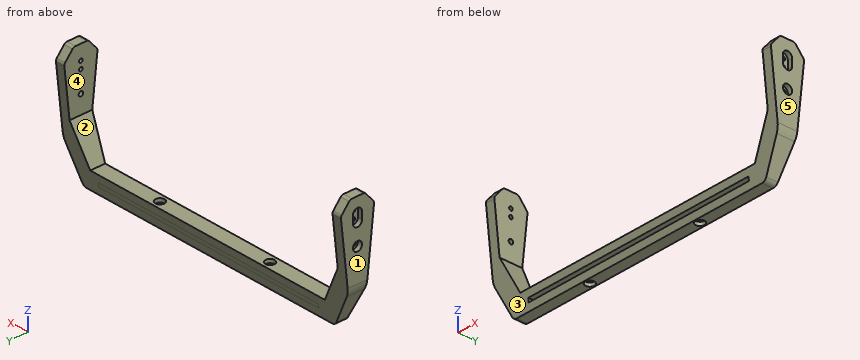
from build123d import *
from OCP.BRepFilletAPI import BRepFilletAPI_MakeChamfer

# Parameters (mm, degrees)
SKETCH4_R                       = 1
SKETCH4_R_2                     = 0.9999999999999998
SKETCH4_R_3                     = 1.250000000000001
BOSS_EXTRUDE1_DEPTH             = 5
BOSS_EXTRUDE2_START             = -79.75
BOSS_EXTRUDE2_DEPTH             = 159.5
BOSS_EXTRUDE3_REACH             = 103.717
SKETCH6_W                       = 14.25
SKETCH6_H                       = 2.1000000000000014
BOSS_EXTRUDE3_DIRECTION_2_REACH = 103.717
SKETCH11_R                      = 0.9999999999999983
CUT_EXTRUDE4_DEPTH              = 101.58679916039975
SKETCH12_R                      = 2.4999999999999982
SKETCH12_R_2                    = 2.500000000000002
CUT_EXTRUDE5_DEPTH              = 2
CUT_EXTRUDE6_START              = -2
SKETCH13_R                      = 2.4999999999999982
SKETCH13_R_2                    = 2.500000000000002
CUT_EXTRUDE6_DEPTH              = 2
CHAMFER3_SIZE                   = 10
CHAMFER3_SIZE2                  = 20
CHAMFER4_SIZE                   = 20
CHAMFER4_SIZE2                  = 10
BOSS_EXTRUDE4_START             = -65.5
BOSS_EXTRUDE4_DEPTH             = 131
SKETCH15_R                      = 2.4999999999999982
CUT_EXTRUDE7_DEPTH              = 2.5
FILLET1_R                       = 2
FILLET2_R                       = 10
FILLET3_R                       = 3


# Read off the part's stored shape, not the designer's step: Boss-Extrude4
with BuildPart() as part:
    # Sketch4 → Boss-Extrude1 (new body)
    with BuildSketch(Plane(origin=(79.75, 0, 0), x_dir=(0, 0, -1), z_dir=(1, 0, 0))):
        Polygon((-7.999999999999998, 4), (-7.999999999999998, -4), (-1.87164445504816, -9.142300877492296), (55.5, -3), (55.5, 3), (-1.8716444550481652, 9.142300877492302), align=None)
        Circle(SKETCH4_R, mode=Mode.SUBTRACT)
        with Locations((4, 0)):
            Circle(SKETCH4_R_2, mode=Mode.SUBTRACT)
        with Locations((15.5, 0)):
            Circle(SKETCH4_R_3, mode=Mode.SUBTRACT)
    extrude(amount=BOSS_EXTRUDE1_DEPTH)


with BuildPart() as body_2:
    # Mirror1: mirrored copy
    add(part.part.mirror(Plane(origin=(0, 0, 0), x_dir=(0, 0, 1), z_dir=(1, 0, 0))))


with BuildPart() as part_1:
    add(part.part)

    add(body_2.part)  # Boss-Extrude2 merges body 2
    # Sketch5 → Boss-Extrude2 (add)
    with BuildSketch(Plane(origin=(0, 0, 0), x_dir=(0, 0, -1), z_dir=(1, 0, 0)).offset(BOSS_EXTRUDE2_START)):
        Polygon((51.49999999999999, 3.428246457694266), (51.49999999999999, -3.428246457694267), (55.5, -3), (55.5, 3), align=None)
        Polygon((45.4, 4.081322305678019), (45.4, -4.081322305678019), (49.39999999999999, -3.6530758479837546), (49.39999999999999, 3.6530758479837546), align=None)
    extrude(amount=BOSS_EXTRUDE2_DEPTH)

    # Boss-Extrude3: up to this plane
    boss_extrude3_end = Plane(origin=(84.75, 3, -55.5), z_dir=(0, -0.9943177075979668, 0.10645325902537786))
    # Sketch6 → Boss-Extrude3 (add, up to the surface)
    with BuildSketch(Plane(origin=(0, 0, 0), x_dir=(1, 0, 0), z_dir=(0, 1, 0)), mode=Mode.PRIVATE) as boss_extrude3_sk1:
        with Locations((-72.625, 50.44999999999999)):
            Rectangle(SKETCH6_W, SKETCH6_H)
    boss_extrude3_tool1 = split(extrude(boss_extrude3_sk1.sketch, amount=BOSS_EXTRUDE3_REACH, mode=Mode.PRIVATE), bisect_by=boss_extrude3_end, keep=Keep.BOTH, mode=Mode.PRIVATE)
    add(boss_extrude3_tool1.solids().sort_by_distance((-72.625, 0, -50.45))[0])
    # Sketch6 → Boss-Extrude3 (add, up to the surface)
    with BuildSketch(Plane(origin=(0, 0, 0), x_dir=(1, 0, 0), z_dir=(0, 1, 0)), mode=Mode.PRIVATE) as boss_extrude3_sk2:
        Polygon((65.5, 49.400000000000006), (79.75, 49.39999999999999), (79.75, 51.49999999999999), (65.5, 51.50000000000001), align=None)
    boss_extrude3_tool2 = split(extrude(boss_extrude3_sk2.sketch, amount=BOSS_EXTRUDE3_REACH, mode=Mode.PRIVATE), bisect_by=boss_extrude3_end, keep=Keep.BOTH, mode=Mode.PRIVATE)
    add(boss_extrude3_tool2.solids().sort_by_distance((72.625, 0, -50.45))[0])

    # Boss-Extrude3 direction 2: up to this plane
    boss_extrude3_direction_2_end = Plane(origin=(84.75, -9.142300877492296, 1.87164445504816), z_dir=(0, 0.9943177075979668, 0.10645325902537779))
    # Sketch6 → Boss-Extrude3 direction 2 (add, up to the surface)
    with BuildSketch(Plane(origin=(0, 0, 0), x_dir=(1, 0, 0), z_dir=(0, 1, 0)), mode=Mode.PRIVATE) as boss_extrude3_direction_2_sk1:
        with Locations((-72.625, 50.44999999999999)):
            Rectangle(SKETCH6_W, SKETCH6_H)
    boss_extrude3_direction_2_tool1 = split(extrude(boss_extrude3_direction_2_sk1.sketch, amount=-BOSS_EXTRUDE3_DIRECTION_2_REACH, mode=Mode.PRIVATE), bisect_by=boss_extrude3_direction_2_end, keep=Keep.BOTH, mode=Mode.PRIVATE)
    add(boss_extrude3_direction_2_tool1.solids().sort_by_distance((-72.625, 0, -50.45))[0])
    # Sketch6 → Boss-Extrude3 direction 2 (add, up to the surface)
    with BuildSketch(Plane(origin=(0, 0, 0), x_dir=(1, 0, 0), z_dir=(0, 1, 0)), mode=Mode.PRIVATE) as boss_extrude3_direction_2_sk2:
        Polygon((65.5, 49.400000000000006), (79.75, 49.39999999999999), (79.75, 51.49999999999999), (65.5, 51.50000000000001), align=None)
    boss_extrude3_direction_2_tool2 = split(extrude(boss_extrude3_direction_2_sk2.sketch, amount=-BOSS_EXTRUDE3_DIRECTION_2_REACH, mode=Mode.PRIVATE), bisect_by=boss_extrude3_direction_2_end, keep=Keep.BOTH, mode=Mode.PRIVATE)
    add(boss_extrude3_direction_2_tool2.solids().sort_by_distance((72.625, 0, -50.45))[0])

    # Sketch11 → Cut-Extrude4 (cut, through all)
    with BuildSketch(Plane.XY.offset(-45.4)):
        with Locations((-32.75, -1.61e-15)):
            Circle(SKETCH11_R)
        with Locations((32.75, 2.4e-15)):
            Circle(SKETCH11_R)
    extrude(amount=-CUT_EXTRUDE4_DEPTH, mode=Mode.SUBTRACT)

    # Sketch12 → Cut-Extrude5 (cut)
    with BuildSketch(Plane.XY.offset(-45.4)):
        with Locations((-32.75, -1.73e-15)):
            Circle(SKETCH12_R)
        with Locations((32.75, 3.47e-15)):
            Circle(SKETCH12_R_2)
    extrude(amount=-CUT_EXTRUDE5_DEPTH, mode=Mode.SUBTRACT)

    # Sketch13 → Cut-Extrude6 (cut)
    with BuildSketch(Plane(origin=(0, 0, -55.5), x_dir=(-1, 0, 0), z_dir=(0, 0, -1)).offset(CUT_EXTRUDE6_START)):
        with Locations(Location((-32.75, 3.47e-15, 0), (0, 0, 180))):
            Circle(SKETCH13_R)
        with Locations(Location((32.75, 0, 0), (0, 0, 180))):
            Circle(SKETCH13_R_2)
    extrude(amount=CUT_EXTRUDE6_DEPTH, mode=Mode.SUBTRACT)

    # Chamfer3: one chamfer whose edges measure the first distance from different faces: ONE call of the kernel's chamfer builder (chamfer() names one face for all edges)
    chamfer3_edges_1 = [part_1.edges().sort_by_distance(p)[0] for p in [
        (84.75, 0, -55.5),
    ]]
    chamfer3_side_1 = [part_1.faces().sort_by_distance(p)[0] for p in [
        (6.55e-15, -1.2e-16, -55.5),
    ]]
    chamfer3_edges_2 = [part_1.edges().sort_by_distance(p)[0] for p in [
        (79.75, 0, -45.4),
    ]]
    chamfer3_side_2 = [part_1.faces().sort_by_distance(p)[0] for p in [
        (3.3e-16, 1.1e-16, -45.4),
    ]]
    chamfer3 = BRepFilletAPI_MakeChamfer(part_1.part.solid().wrapped)
    for e in chamfer3_edges_1:
        chamfer3.Add(CHAMFER3_SIZE, CHAMFER3_SIZE2, e.wrapped, chamfer3_side_1[0].wrapped)  # the first distance lies on this face
    for e in chamfer3_edges_2:
        chamfer3.Add(CHAMFER3_SIZE, CHAMFER3_SIZE2, e.wrapped, chamfer3_side_2[0].wrapped)  # the first distance lies on this face
    add(Compound.cast(chamfer3.Shape()), mode=Mode.REPLACE)

    # Chamfer4: one chamfer whose edges measure the first distance from different faces: ONE call of the kernel's chamfer builder (chamfer() names one face for all edges)
    chamfer4_edges_1 = [part_1.edges().sort_by_distance(p)[0] for p in [
        (-79.75, 0, -45.4),
    ]]
    chamfer4_side_1 = [part_1.faces().sort_by_distance(p)[0] for p in [
        (-79.75, 6.138766924124398, 4.573009379877834),
    ]]
    chamfer4_edges_2 = [part_1.edges().sort_by_distance(p)[0] for p in [
        (-84.75, 0, -55.5),
    ]]
    chamfer4_side_2 = [part_1.faces().sort_by_distance(p)[0] for p in [
        (-84.75, 2.08e-15, -19.394723563601886),
    ]]
    chamfer4 = BRepFilletAPI_MakeChamfer(part_1.part.solid().wrapped)
    for e in chamfer4_edges_1:
        chamfer4.Add(CHAMFER4_SIZE, CHAMFER4_SIZE2, e.wrapped, chamfer4_side_1[0].wrapped)  # the first distance lies on this face
    for e in chamfer4_edges_2:
        chamfer4.Add(CHAMFER4_SIZE, CHAMFER4_SIZE2, e.wrapped, chamfer4_side_2[0].wrapped)  # the first distance lies on this face
    add(Compound.cast(chamfer4.Shape()), mode=Mode.REPLACE)

    # Boss-Extrude4 outline → Boss-Extrude4 (add)
    with BuildSketch(Plane.YZ.offset(BOSS_EXTRUDE4_START)):
        Polygon((3.428246458, -51.5), (3.653075848, -49.4), (2.5, -49.4), (2.5, -51.5), align=None)
    extrude(amount=BOSS_EXTRUDE4_DEPTH)

    # Sketch15 → Cut-Extrude7 (cut)
    with BuildSketch(Plane(origin=(84.75, 0, 0), x_dir=(0, 0, -1), z_dir=(1, 0, 0))):
        with Locations((15.5, 0)):
            Circle(SKETCH15_R)
        with BuildLine():
            Line((4, 2.5), (0, 2.5))
            ThreePointArc((0, 2.5), (-2.5, 3.1e-16), (0, -2.5))
            Line((0, -2.5), (4, -2.5))
            ThreePointArc((4, -2.5), (6.5, 0), (4, 2.5))
        make_face()
    cut_extrude7 = extrude(amount=-CUT_EXTRUDE7_DEPTH, mode=Mode.SUBTRACT)

    # Mirror2: Cut-Extrude7 across plane
    add(cut_extrude7.mirror(Plane(origin=(0, 0, 0), x_dir=(0, 0, 1), z_dir=(1, 0, 0))), mode=Mode.SUBTRACT)

    # Fillet1
    fillet1_edges = [part_1.edges().sort_by_distance(p)[0] for p in [
        (82.25, 9.142300877492302, 1.8716444550481652),
        (82.25, -9.142300877492296, 1.87164445504816),
        (82.25, -4, 7.999999999999998),
        (82.25, 4, 7.999999999999998),
        (-82.25, 4, 7.999999999999998),
        (-82.25, -4, 7.999999999999998),
        (-82.25, -9.142300877492296, 1.87164445504816),
        (-82.25, 9.142300877492302, 1.8716444550481652),
    ]]
    fillet(fillet1_edges, radius=FILLET1_R)

    # Fillet2
    fillet2_edges = [part_1.edges().sort_by_distance(p)[0] for p in [
        (84.75, 8.9e-16, -35.5),
        (-84.75, 8.9e-16, -35.5),
    ]]
    fillet(fillet2_edges, radius=FILLET2_R)

    # Fillet3
    fillet3_edges = [part_1.edges().sort_by_distance(p)[0] for p in [
        (74.75, 0, -55.5),
        (-74.75, 0, -55.5),
    ]]
    fillet(fillet3_edges, radius=FILLET3_R)


solid = part_1.part
Design review of the part built by this model. Coordinates are the model's own, in mm. Face numbers are marked on the shaded views. A direction names the side the tool comes from. Round coordinates to 2 decimals unless told otherwise and drop trailing zeros. Loops run counter-clockwise (first coordinate to the right, second up) from the corner with the lowest first, then second, coordinate; pieces in that order, holes last. Notation, with made-up numbers: (68.5, 3) - (123.5, 3) arc R20 cw to (123.5, 20) - close; hole circle Ø11 at (41, 48.5). An arc over 180 degrees is marked (long way). One line per item, written item: value. Start each with the question number.
1) Insertion check: pin 1 Ø1.2 at (x, y) = (32.75, 0) entering from +Z; pin 2 Ø5.5 at (x, y) = (-34, 0) entering from -Z; pin 3 Ø2.5 at (x, y) = (20.5, 0) entering from +Z; pin 4 Ø3 at (x, y) = (-32.75, 0) entering from +Z. Each pin has a flat end and moves straight along its axis. Give the tip position at first contact, or say it passes through.
2) Draft analysis for pull direction X (two halves, no side actions). For the marked faces 1, 2 and 3, state which applies: +X half, -X half, draft (parallel to the pull), parting line (faces both ways), or undercut.
3) Consider section A-A on x = 4.5. Give the boundary of the cut face in (y, z), then the cut area to 3 significant figures.
4) Consider section C-C on z = -28.5. Give the boundary of the cut face in (x, y), then the cut area to 3 significant figures.
5) To check wall thickness, follow L1, parallel to X at y = -8, z = -8; L2, parallel to X at y = -1.5, z = 0.5; L3, parallel to Z at x = 81, y = 0. State the ranges of each line that lie inside material, in increasing order. Write a range as from..to.
6) For the marked faces 4 and 5, list the 3-axis set-ups (+Z, -Z, +X, -X, +Y, -Y) from which the entire face can be reached by the end or side of a thin tool; tool diameter is ignored.
7) Consider section B-B on z = -22. Give the boundary of the cut face in (x, y).
Reported:
1. pin 1: passes through
1. pin 2: stops at z = -55.5
1. pin 3: stops at z = -45.4
1. pin 4: stops at z = -47.4
2. face 1: -X half
2. face 2: undercut
2. face 3: draft
3. outline: (-4.08, -45.4) - (-3.65, -49.4) - (2.5, -49.4) - (2.5, -51.5) - (-3.43, -51.5) - (-3, -55.5) - (3, -55.5) - (4.08, -45.4) - close
3. area: 58.8 mm^2
4. outline: (-84.75, -5.89) - (-78.2, -5.89) - (-78.2, 5.89) - (-84.75, 5.89) - close; (78.2, -5.89) - (84.75, -5.89) - (84.75, 5.89) - (78.2, 5.89) - close
4. area: 154 mm^2
5. L1: x = -84.75..-79.75, 79.75..84.75
5. L2: x = -82.25..-79.75, 79.75..82.25
5. L3: z = -43..-16.75, -14.25..-5, -3..-1, 1..8
6. face 4: +Z, +Y, -Y
6. face 5: +Z, -Z, +X, +Y, -Y
7. outline: (-84.75, -6.59) - (-79.75, -6.59) - (-79.75, 6.59) - (-84.75, 6.59) - close; (79.75, -6.59) - (84.75, -6.59) - (84.75, 6.59) - (79.75, 6.59) - close
